Part model, mm, in its own coordinate system. Round coordinates to 2 decimals unless told otherwise and drop trailing zeros. Write each loop counter-clockwise with the first axis right and the second up, starting at its lowest first coordinate (ties: lowest second). Pieces come first, ordered by that corner, then holes.
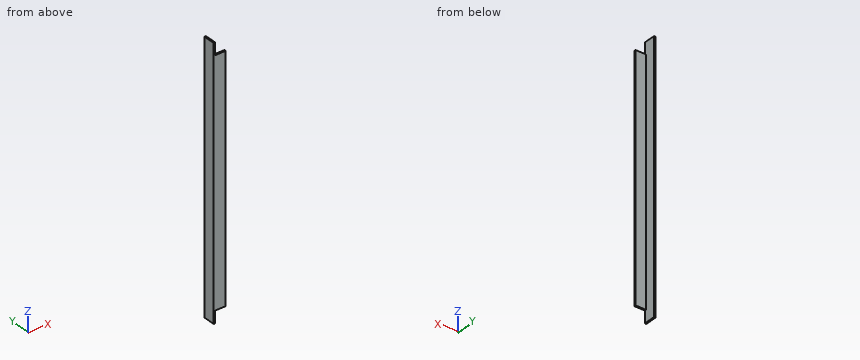
Autodesk Inventor part; units mm, degrees
ref_plane "YZ Plane" through (0, 0, 0) normal (1, 0, 0) x (0, 1, 0)
ref_plane "XZ Plane" through (0, 0, 0) normal (0, 1, 0) x (-1, 0, 0)
ref_plane "XY Plane" through (0, 0, 0) normal (0, 0, 1) x (1, 0, 0)
sketch "Sketch1" plane through (0, 0, 0) normal (0, 0, 1) x (1, 0, 0)
  line L0 (0, 0) -> (0, 25.4)
  line L1 (0, 0) -> (25.4, 0)
  line L2 (25.4, 3.175) -> (3.175, 3.175)
  line L3 (3.175, 3.175) -> (3.175, 25.4)
  line L4 (25.4, 3.175) -> (25.4, 0)
  line L5 (0, 25.4) -> (3.175, 25.4)
  dimension "d0" = 25.4
  dimension "d1" = 25.4
  dimension "d2" = 3.175
extrude "Extrusion1" add sketch "Sketch1" along normal blind 558.8
sketch "Sketch2" plane through (3.175, 3.175, 0) normal (0, 1, 0) x (1, 0, 0)
  line L0 (0, 0) -> (0, -558.8)
  line L1 (0, -25.4) -> (22.225, -25.4)
  line L2 (22.225, 0) -> (22.225, -558.8)
  line L3 (0, -533.4) -> (22.225, -533.4)
  line L4 (22.225, -558.8) -> (0, -558.8)
  line L5 (0, 0) -> (22.225, 0)
  line L6 (22.225, -533.4) -> (22.225, -558.8)
  line L7 (0, -558.8) -> (0, -533.4)
  line L8 (-3.175, -558.8) -> (22.225, -558.8)
  line L9 (0, -25.4) -> (0, 0)
  line L10 (-3.175, 0) -> (-3.175, -558.8)
  line L11 (22.225, 0) -> (-3.175, 0)
  line L12 (0, 0) -> (22.225, 0)
  line L13 (22.225, 0) -> (22.225, -25.4)
  line L14 (0, -558.8) -> (22.225, -558.8)
  dimension "d5" = 25.4
  dimension "d6" = 25.4
extrude "Extrusion2" cut sketch "Sketch2" against normal blind 25.4 contours L5 L2 L1 L0 | L3 L2 L4 L0
properties part number "22 cut 20 L bracket"
Q1. Wall check: line 1 (X direction, y = 24.5, z = 402.5) (3 decimals). Give the ranges that are in metal, low to high.
Q2. Saw through at C-C, the plane x = 11.75. Write the cut outline in (y, z) (3 decimals).
Q3. Saw through at B-B, the plane y = 10.25. Write the cut outline in (x, z) (3 decimals).
Q4. Saw through at A-A, the plane z = 193. Write the cut outline in (x, y) (3 decimals), and give its area (3 significant figures).
Q5. Drop flat-ended pins along their axis: P1, Ø5, axis at x = 11.5, y = 7, coming from the +Z side; P2, Ø5, axis at x = 17, z = 272, coming from the +Y side (3 decimals); P3, Ø5, axis at x = 13.5, y = 4.5, coming from the +Z side; P4, Ø7.5, axis at y = 18, z = 232.5, coming from the +X side (3 decimals). Give the stop position or say it passes through.
Computed:
1. line 1: x = 0 to 3.175
2. outline: (0, 25.4) - (3.175, 25.4) - (3.175, 533.4) - (0, 533.4) - close
3. outline: (0, 0) - (3.175, 0) - (3.175, 558.8) - (0, 558.8) - close
4. outline: (0, 0) - (25.4, 0) - (25.4, 3.175) - (3.175, 3.175) - (3.175, 25.4) - (0, 25.4) - close
4. area: 151 mm2
5. P1: passes through
5. P2: stops at y = 3.175
5. P3: stops at z = 533.4
5. P4: stops at x = 3.175
